Source: three-view drawing plus pictorial views. Frame: mm from the lowest corner of the part. Give positions to 0.01 mm unless a question says otherwise; leave off trailing zeros. Order: outer loops, then holes, each group sorted by start corner. A loop starts at its lowest first (then second) coordinate and runs counter-clockwise, first axis right, second up. Notation, with made-up numbers: (66, 88) - (96, 88) arc R33 cw to (96, 117) - close; hole circle Ø5 at (84, 43.5). An arc over 180 degrees is marked (long way). Use one line per item in the form item = value.
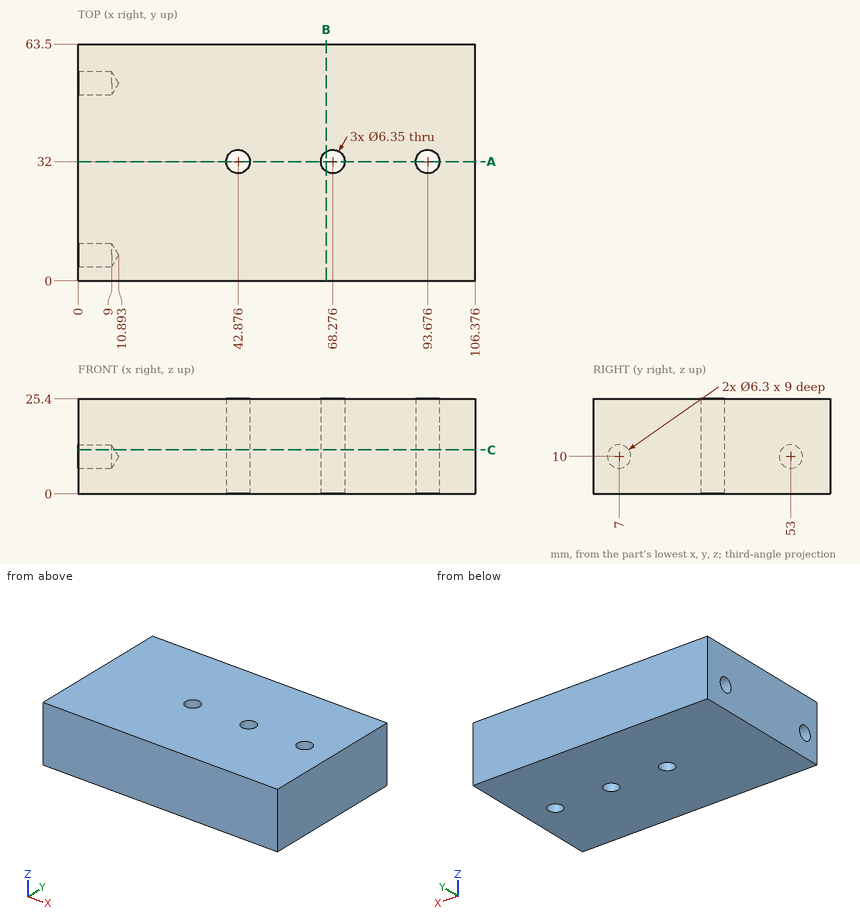
(1) Contact query for a flat-ended pin moving along its axis: pin 1 Ø4 at (x, y) = (42.88, 32) entering from +Z. Output: stop coordinate, or through.
Computed values:
pin_1 = through
(2) Cut plane B-B on x = 66.5. Output: boundary loops of the cut face in (y, z), plus the area to 3 significant figures.
Computed values:
outline = (0, 0) - (29.37, 0) - (29.37, 25.4) - (0, 25.4) - close; (34.63, 0) - (63.5, 0) - (63.5, 25.4) - (34.63, 25.4) - close
area = 1,480 mm²
(3) Cut plane C-C on z = 11.75. Give the number of separate pieces and of enclosed holes in the cut face, plus the area to 3 significant figures.
Computed values:
separate_pieces = 1
enclosed_holes = 3
area = 6,560 mm²
(4) Ray query, line 1 along Y through (x, z) = (4.5, 10); line 2 along Z through (x, y) = (5.5, 7); line 3 along X through (y, z) = (30, 12.5) (1 decimal). Return the intervals inside material, ascending.
Computed values:
line_1 = 0 to 3.85, 10.15 to 49.85, 56.15 to 63.5
line_2 = 0 to 6.85, 13.15 to 25.4
line_3 = 0 to 40.4, 45.3 to 65.8, 70.7 to 91.2, 96.1 to 106.4
(5) Cut plane A-A on y = 32. Output: boundary loops of the cut face in (x, z), plus the area to 3 significant figures.
Computed values:
outline = (0, 0) - (39.7, 0) - (39.7, 25.4) - (0, 25.4) - close; (46.05, 0) - (65.1, 0) - (65.1, 25.4) - (46.05, 25.4) - close; (71.45, 0) - (90.5, 0) - (90.5, 25.4) - (71.45, 25.4) - close; (96.85, 0) - (106.38, 0) - (106.38, 25.4) - (96.85, 25.4) - close
area = 2,220 mm²
